Can you work these out from the model? Positions are in its coordinate system, mm. Face numbers are marked on the shaded views. A direction names the side the tool comes from. Give positions to 0.01 mm unless a question says otherwise; leave off trailing zeros. Loops run counter-clockwise (first coordinate to the right, second up) from the corner with the lowest first, then second, coordinate; pieces in that order, holes last. Notation, with made-up numbers: (65.25, 22.5) - (104.25, 22.5) arc R28 cw to (104.25, 61.5) - close; hole circle Ø9 at (-18.5, -35). An arc over 180 degrees is marked (long way). Answer as a JSON object with one key per item and string values. Group by question number.
Item 1: Please list where these lines run through material, in increasing order: L1, parallel to X at y = 2, z = 41.5; L2, parallel to Y at x = 20, z = 10.
Item 2: Suppose I cut it at D-D on y = -28. Write out the boundary of the cut face in (x, z).
Item 3: Suppose I cut it at B-B on x = -8. Write out the boundary of the cut face in (y, z), and give its area (3 significant figures).
Item 4: Will this pin go through, and if not, where does the flat tip stop? pin 1 (7 mm diameter, centred on x = -9.5, y = -35.5, fed in from +Z).
Item 5: Thinking about a two-plate mould opening in X: for the marked faces 1, 2 and 3, which applies, pulls with the +X half, pulls with the -X half, needs draft (parallel to the pull), parting line crosses it, or undercut?
Item 6: Suppose I cut it at A-A on z = 31.75. Write out the boundary of the cut face in (x, y).
Item 7: Which directions (+Z, -Z, +X, -X, +Y, -Y) give clear straight access to the entire face, cutting with the end or side of a thin tool? Please do the marked faces 4 and 5.
Item 8: Suppose I cut it at C-C on y = 0. Write out the boundary of the cut face in (x, z).
from build123d import *

# Parameters (mm, degrees)
F0_W     = 152.4
F0_H     = 76.2
F0_W_2   = 139.7
F0_H_2   = 63.5
F1_DEPTH = 63.5
F2_W     = 50.8
F2_H     = 25.4
F3_DEPTH = 81.026
F4_R     = 6.35
F5_DEPTH = 156.972


with BuildPart() as f1:
    # F0 (on Top) → F1 (new body)
    with BuildSketch(Plane.XY):
        Rectangle(F0_W, F0_H)
        Rectangle(F0_W_2, F0_H_2, mode=Mode.SUBTRACT)
    extrude(amount=F1_DEPTH)

    # F2 (on face) → F3 (cut)
    with BuildSketch(Plane.XZ.offset(38.1)):
        with Locations((0, 50.8)):
            Rectangle(F2_W, F2_H)
    extrude(amount=-F3_DEPTH, mode=Mode.SUBTRACT)

    # F4 (on face) → F5 (cut)
    with BuildSketch(Plane.YZ.offset(76.2)):
        with Locations((0, 31.75)):
            Circle(F4_R)
    extrude(amount=-F5_DEPTH, mode=Mode.SUBTRACT)


solid = f1.part
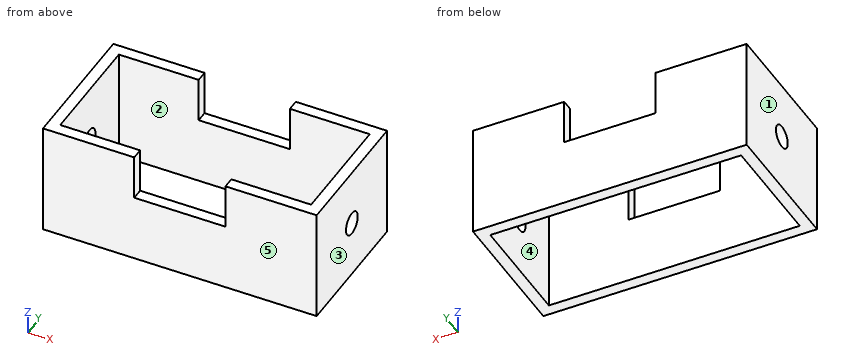
Worked out:
{
 "1": {"L1": "x = -76.2 to -69.85, 69.85 to 76.2", "L2": "y = -38.1 to -31.75, 31.75 to 38.1"},
 "2": {"outline": "(-76.2, 0) - (-69.85, 0) - (-69.85, 63.5) - (-76.2, 63.5) - close; (69.85, 0) - (76.2, 0) - (76.2, 63.5) - (69.85, 63.5) - close"},
 "3": {"outline": "(-38.1, 0) - (-31.75, 0) - (-31.75, 38.1) - (-38.1, 38.1) - close; (31.75, 0) - (38.1, 0) - (38.1, 38.1) - (31.75, 38.1) - close", "area": "484 mm2"},
 "4": {"pin 1": "stops at z = 38.1"},
 "5": {"face 1": "pulls with the -X half", "face 2": "undercut", "face 3": "pulls with the +X half"},
 "6": {"outline": "(-76.2, -38.1) - (76.2, -38.1) - (76.2, -6.35) - (69.85, -6.35) - (69.85, -31.75) - (-69.85, -31.75) - (-69.85, -6.35) - (-76.2, -6.35) - close; (-76.2, 6.35) - (-69.85, 6.35) - (-69.85, 31.75) - (69.85, 31.75) - (69.85, 6.35) - (76.2, 6.35) - (76.2, 38.1) - (-76.2, 38.1) - close"},
 "7": {"face 4": "+Z, -Z", "face 5": "+Z, -Z, +X, -X, -Y"},
 "8": {"outline": "(-76.2, 0) - (-69.85, 0) - (-69.85, 25.4) - (-76.2, 25.4) - close; (-76.2, 38.1) - (-69.85, 38.1) - (-69.85, 63.5) - (-76.2, 63.5) - close; (69.85, 0) - (76.2, 0) - (76.2, 25.4) - (69.85, 25.4) - close; (69.85, 38.1) - (76.2, 38.1) - (76.2, 63.5) - (69.85, 63.5) - close"}
}
